Can you work these out from the drawing? Everything is in mm from the part's minimum corner. Coordinates: 2 decimals unless noted, no trailing zeros. Order: outer loops, then holes, each group sorted by start corner. A loop starts at its lowest first (then second) coordinate and runs counter-clockwise, first axis right, second up. Notation, with made-up numbers: M 6,-34 L 27,-34 A16 cw 27,-23 Z; hole C 58,-19.5 d7. An arc over 180 degrees is marked long. Answer as a JSON object with one key per item and string values.
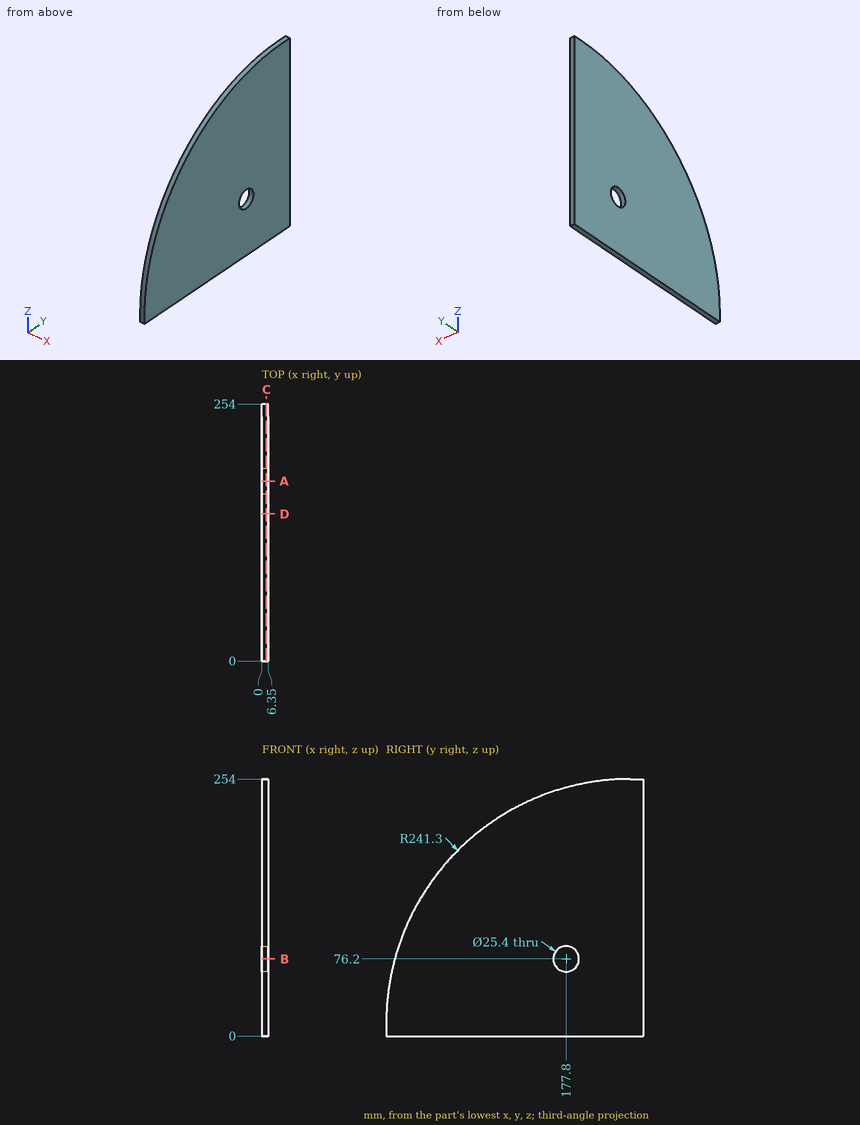
Item 1: I want a section at D-D, the plane y = 145.5. Write out the boundary of the cut face in (x, z).
Answers follow:
{"outline": "M 0,0 L 6.35,0 L 6.35,234.17 L 0,234.17 Z"}
Item 2: I want a section at A-A, the plane y = 177.8. Write out the boundary of the cut face in (x, z).
Answers follow:
{"outline": "M 0,0 L 6.35,0 L 6.35,63.5 L 0,63.5 Z; M 0,88.9 L 6.35,88.9 L 6.35,245.49 L 0,245.49 Z"}
Item 3: I want a section at C-C, the plane x = 4.5. Write out the boundary of the cut face in (y, z).
Answers follow:
{"outline": "M 0,0 L 254,0 L 254,254 L 241.3,254 A241.3 ccw 0,12.7 Z; hole C 177.8,76.2 d25.4"}
Item 4: Please list where these lines run through material, in increasing order: line 1 (Y direction, x = 3, z = 68); line 2 (Y direction, x = 3, z = 78.5); line 3 (Z direction, x = 0.5, y = 241).
Answers follow:
{"line 1": "y = 6.42 to 168.1, 187.5 to 254", "line 2": "y = 9.14 to 165.31, 190.29 to 254", "line 3": "z = 0 to 254"}
Item 5: I'm going to push flat-ended pins straight in: pin 1 (10 mm diameter, centred on y = 119, z = 183.5, fed in from -X); pin 2 (1.5 mm diameter, centred on x = 2.5, y = 136, fed in from +Z); pin 3 (1.5 mm diameter, centred on x = 3, y = 120, fed in from +Z); pin 4 (3 mm diameter, centred on x = 4.5, z = 125, fed in from -Y). Where does each tip first touch, or does it pass through?
Answers follow:
{"pin 1": "stops at x = 0", "pin 2": "stops at z = 230.17", "pin 3": "stops at z = 221.73", "pin 4": "stops at y = 26.94"}
Item 6: I want a section at B-B, the plane z = 76.2. Write out the boundary of the cut face in (x, y), plus the area to 3 significant figures.
Answers follow:
{"outline": "M 0,8.51 L 6.35,8.51 L 6.35,165.1 L 0,165.1 Z; M 0,190.5 L 6.35,190.5 L 6.35,254 L 0,254 Z", "area": "1,400 mm^2"}
